```python
from build123d import *

# Parameters (mm, degrees)
BOSS_EXTRUDE1_DEPTH = 10
SKETCH2_R           = 3
SKETCH2_R_2         = 1.75
CUT_EXTRUDE1_DEPTH  = 3
SKETCH2_5_R         = 1.75
CUT_EXTRUDE2_DEPTH  = 58.445626465
SKETCH5_R           = 19
CUT_EXTRUDE3_DEPTH  = 58.445626465


with BuildPart() as part:
    # Sketch1 → Boss-Extrude1 (new body)
    with BuildSketch(Plane(origin=(0, 0, 0), x_dir=(1, 0, 0), z_dir=(0, 1, 0))):
        with BuildLine():
            Line((4, 0), (36, 0))
            ThreePointArc((36, 0), (38.828427125, 1.171572875), (40, 4))
            Line((40, 4), (40, 36))
            ThreePointArc((40, 36), (38.828427125, 38.828427125), (36, 40))
            Line((36, 40), (4, 40))
            ThreePointArc((4, 40), (1.171572875, 38.828427125), (0, 36))
            Line((0, 36), (0, 4))
            ThreePointArc((0, 4), (1.171572875, 1.171572875), (4, 0))
        make_face()
    extrude(amount=BOSS_EXTRUDE1_DEPTH)

    # Sketch2 → Cut-Extrude1 (cut)
    # profile 1 of 8: a face of its own
    with BuildSketch(Plane(origin=(0, 10, 0), x_dir=(1, 0, 0), z_dir=(0, 1, 0))):
        with Locations(Location((36, 36, 0), (0, 0, 270))):
            Circle(SKETCH2_R)
        with Locations((36, 36)):
            Circle(SKETCH2_R_2, mode=Mode.SUBTRACT)
    # profile 2 of 8: a face of its own
    with BuildSketch(Plane(origin=(0, 10, 0), x_dir=(1, 0, 0), z_dir=(0, 1, 0))):
        with Locations((36, 36)):
            Circle(SKETCH2_R_2)
    # profile 3 of 8: a face of its own
    with BuildSketch(Plane(origin=(0, 10, 0), x_dir=(1, 0, 0), z_dir=(0, 1, 0))):
        with Locations(Location((4, 36, 0), (0, 0, 270))):
            Circle(SKETCH2_R)
        with Locations((4, 36)):
            Circle(SKETCH2_R_2, mode=Mode.SUBTRACT)
    # profile 4 of 8: a face of its own
    with BuildSketch(Plane(origin=(0, 10, 0), x_dir=(1, 0, 0), z_dir=(0, 1, 0))):
        with Locations((4, 36)):
            Circle(SKETCH2_R_2)
    # profile 5 of 8: a face of its own
    with BuildSketch(Plane(origin=(0, 10, 0), x_dir=(1, 0, 0), z_dir=(0, 1, 0))):
        with Locations(Location((4, 4, 0), (0, 0, 270))):
            Circle(SKETCH2_R)
        with Locations((4, 4)):
            Circle(SKETCH2_R_2, mode=Mode.SUBTRACT)
    # profile 6 of 8: a face of its own
    with BuildSketch(Plane(origin=(0, 10, 0), x_dir=(1, 0, 0), z_dir=(0, 1, 0))):
        with Locations((4, 4)):
            Circle(SKETCH2_R_2)
    # profile 7 of 8: a face of its own
    with BuildSketch(Plane(origin=(0, 10, 0), x_dir=(1, 0, 0), z_dir=(0, 1, 0))):
        with Locations(Location((36, 4, 0), (0, 0, 270))):
            Circle(SKETCH2_R)
        with Locations((36, 4)):
            Circle(SKETCH2_R_2, mode=Mode.SUBTRACT)
    # profile 8 of 8: a face of its own
    with BuildSketch(Plane(origin=(0, 10, 0), x_dir=(1, 0, 0), z_dir=(0, 1, 0))):
        with Locations((36, 4)):
            Circle(SKETCH2_R_2)
    extrude(amount=-CUT_EXTRUDE1_DEPTH, mode=Mode.SUBTRACT)

    # Sketch2_5 → Cut-Extrude2 (cut, through all)
    with BuildSketch(Plane(origin=(0, 10, 0), x_dir=(1, 0, 0), z_dir=(0, 1, 0))):
        with Locations(Location((36, 36, 0), (0, 0, 270))):
            Circle(SKETCH2_5_R)
        with Locations(Location((4, 36, 0), (0, 0, 270))):
            Circle(SKETCH2_5_R)
        with Locations(Location((4, 4, 0), (0, 0, 270))):
            Circle(SKETCH2_5_R)
        with Locations(Location((36, 4, 0), (0, 0, 270))):
            Circle(SKETCH2_5_R)
    extrude(amount=-CUT_EXTRUDE2_DEPTH, mode=Mode.SUBTRACT)

    # Sketch5 → Cut-Extrude3 (cut, through all)
    with BuildSketch(Plane(origin=(0, 10, 0), x_dir=(1, 0, 0), z_dir=(0, 1, 0))):
        with Locations(Location((20, 20, 0), (0, 0, 270))):
            Circle(SKETCH5_R)
    extrude(amount=-CUT_EXTRUDE3_DEPTH, mode=Mode.SUBTRACT)


solid = part.part
```
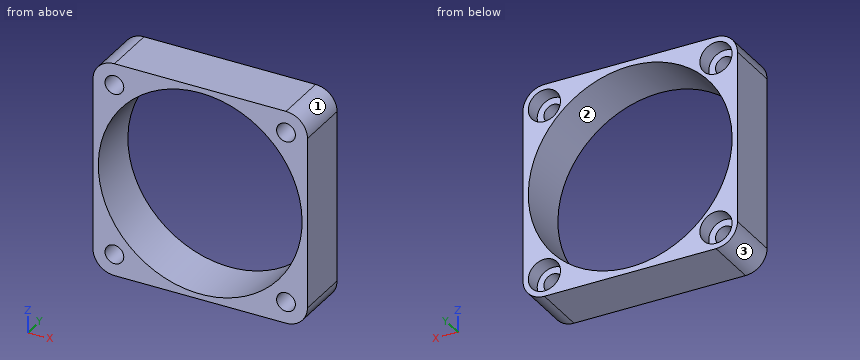
Geometry check sheet. Reference: the model listing, model coordinates, mm. Face numbers are marked on the shaded views. Coordinates: 2 decimals unless noted, no trailing zeros. Loops run counter-clockwise (first coordinate to the right, second up) from the corner with the lowest first, then second, coordinate; pieces in that order, holes last. Notation, with made-up numbers: (64, -30.75) -> (109, -30.75) arc R21 cw to (109, -13.75) -> close; hole circle Ø10 at (30, 88.5). An arc over 180 degrees is marked (long way). Put each result on its own line as item: value.
1) Cross-section at B-B on y = 5. Record the boundary of the cut face in (x, z).
Result set:
outline: (0, -36) arc R4 ccw to (4, -40) -> (36, -40) arc R4 ccw to (40, -36) -> (40, -4) arc R4 ccw to (36, 0) -> (4, 0) arc R4 ccw to (0, -4) -> close; hole circle Ø38 at (20, -20); hole circle Ø3.5 at (4, -36); hole circle Ø3.5 at (4, -4); hole circle Ø3.5 at (36, -36); hole circle Ø3.5 at (36, -4)
2) Gauge pin test, flat ends, axial feed: pin 1 Ø2 at (x, z) = (4, -4) entering from -Y; pin 2 Ø4.5 at (x, z) = (4, -36) entering from +Y. Record the tip position at first contact, or that the pin passes through.
Result set:
pin 1: passes through
pin 2: stops at y = 7
3) Thickness scan on line 1 (X direction, y = 6.75, z = -19.5); line 2 (X direction, y = 7.75, z = -36); line 3 (Z direction, x = 20.5, y = 3.5). Record the ranges inside material, lowest first.
Result set:
line 1: x = 0 to 1.01, 38.99 to 40
line 2: x = 0 to 1, 7 to 9.75, 30.25 to 33, 39 to 40
line 3: z = -40 to -38.99, -1.01 to 0
4) Cross-section at A-A on z = -17. Record the boundary of the cut face in (x, y), plus the area to 3 significant figures.
Result set:
outline: (0, 0) -> (1.24, 0) -> (1.24, 10) -> (0, 10) -> close; (38.76, 0) -> (40, 0) -> (40, 10) -> (38.76, 10) -> close
area: 24.8 mm^2
5) Cross-section at C-C on x = 26.5. Record the boundary of the cut face in (y, z), plus the area to 3 significant figures.
Result set:
outline: (0, -40) -> (10, -40) -> (10, -37.85) -> (0, -37.85) -> close; (0, -2.15) -> (10, -2.15) -> (10, 0) -> (0, 0) -> close
area: 42.9 mm^2
6) Release check for a two-part mould opening along Z. For the marked faces 1, 2 and 3 record: released by +Z, released by -Z, zero draft, split by the parting line, or undercut.
Result set:
face 1: released by +Z
face 2: undercut
face 3: released by -Z
7) Cross-section at D-D on z = -3.5. Record the boundary of the cut face in (x, y), plus the area to 3 significant figures.
Result set:
outline: (0.03, 0) -> (2.32, 0) -> (2.32, 7) -> (1.04, 7) -> (1.04, 10) -> (0.03, 10) -> close; (5.68, 0) -> (10.58, 0) -> (10.58, 10) -> (6.96, 10) -> (6.96, 7) -> (5.68, 7) -> close; (29.42, 0) -> (34.32, 0) -> (34.32, 7) -> (33.04, 7) -> (33.04, 10) -> (29.42, 10) -> close; (37.68, 0) -> (39.97, 0) -> (39.97, 10) -> (38.96, 10) -> (38.96, 7) -> (37.68, 7) -> close
area: 129 mm^2
